Geometry: final body of the model. Coordinates: model frame, mm. A direction names the side the tool comes from. Coordinates: 2 decimals unless noted, no trailing zeros. Order: outer loops, then holes, each group sorted by start corner. A loop starts at its lowest first (then second) coordinate and runs counter-clockwise, first axis right, second up. Notation, with made-up numbers: M -24.5,2.5 L -20.5,2.5 A9 ccw -20.5,17.5 Z; hole C 85,63 d3. An arc over 180 degrees is marked long. Write item = value, one per line. Start each with the question number.
```python
from build123d import *

# Parameters (mm, degrees)
F1_DEPTH = 6.223
F3_DEPTH = 25.4
F4_R     = 5.08
F5_R     = 7.62


with BuildPart() as f1:
    # F0 (on Top) → F1 (new body)
    with BuildSketch(Plane.XY):
        Polygon((-38.1, 0), (0, 0), (38.1, 0), (38.1, 9.5885), (44.45, 9.5885), (44.45, 12.7), (44.45, 15.8115), (38.1, 15.8115), (38.1, 41.3385), (44.45, 41.3385), (44.45, 44.45), (44.45, 47.5615), (38.1, 47.5615), (38.1, 57.15), (0, 57.15), (-38.1, 57.15), (-38.1, 47.5615), (-44.45, 47.5615), (-44.45, 44.45), (-44.45, 41.3385), (-38.1, 41.3385), (-38.1, 15.8115), (-44.45, 15.8115), (-44.45, 12.7), (-44.45, 9.5885), (-38.1, 9.5885), align=None)
    extrude(amount=F1_DEPTH)

    # F2 (on face) → F3 (cut)
    with BuildSketch(Plane.XY.offset(6.223)):
        Polygon((-28.575, 46.0375), (-28.575, 11.1125), (-5.291667, 28.575), align=None)
        Polygon((-24.341667, 50.8), (0, 32.54375), (24.341667, 50.8), align=None)
        Polygon((28.575, 46.0375), (5.291667, 28.575), (28.575, 11.1125), align=None)
        Polygon((24.341667, 6.35), (0, 24.60625), (-24.341667, 6.35), align=None)
    extrude(amount=-F3_DEPTH, mode=Mode.SUBTRACT)

    # F4
    f4_edges = [f1.edges().sort_by_distance(p)[0] for p in [
        (-28.575, 11.1125, 3.1115),
        (-28.575, 46.0375, 3.1115),
        (-5.291667, 28.575, 3.1115),
        (24.341667, 6.35, 3.1115),
        (0, 24.60625, 3.1115),
        (-24.341667, 6.35, 3.1115),
        (28.575, 11.1125, 3.1115),
        (28.575, 46.0375, 3.1115),
        (5.291667, 28.575, 3.1115),
        (0, 32.54375, 3.1115),
        (24.341667, 50.8, 3.1115),
        (-24.341667, 50.8, 3.1115),
    ]]
    fillet(f4_edges, radius=F4_R)

    # F5
    f5_edges = [f1.edges().sort_by_distance(p)[0] for p in [
        (-38.1, 57.15, 3.1115),
        (38.1, 57.15, 3.1115),
        (38.1, 0, 3.1115),
        (-38.1, 0, 3.1115),
    ]]
    fillet(f5_edges, radius=F5_R)


solid = f1.part
```
Item 1: Section query C-C on x = -24. Output: boundary loops of the cut face in (y, z), and give its area (3 significant figures).
Item 2: Reachability of faces 1 (the flat face through (38.1, 28, 3)), 2 (the flat face through (41, 47.562, 3)), 3 (the cylindrical face through (-8.68, 28.51, 3.07)) from +Z, -Z, +X, -X, +Y, -Y: full face, straight path, thin tool, end or side. Return the list, or none.
Item 3: Section query A-A on x = 1.5. Output: boundary loops of the cut face in (y, z), and give its area (3 significant figures).
Item 4: Draft query along X for faces 4 (the cylindrical face through (35.809, 2.173, 3.155)), 5 (the flat face through (41, 9.588, 3)), 6 (the cylindrical face through (0.046, 23.336, 3.068)). Return one class per face: pulls with the +X half, pulls with the -X half, needs draft (parallel to the pull), parting line crosses it, or undercut.
Item 5: Section query D-D on y = 19. Output: boundary loops of the cut face in (x, z) (3 decimals).
Item 6: Material intervals for probe 1 along Y at (x, z) = (-41, 0.5); probe 2 along Y at (x, z) = (2, 3.75); probe 3 along Y at (x, z) = (10, 0.75), sorted ascending. Write a range as [from, to].
Item 7: Section query B-B on y = 30. Output: boundary loops of the cut face in (x, z) (3 decimals), and give its area (3 significant figures).
Item 8: First-contact query: pin 1 (1.5 mm diameter, centred on y = 40.5, z = 1.5, fed in from +X); pin 2 (3 mm diameter, centred on x = -41.5, z = 3, fed in from -Y); pin 3 (3 mm diameter, centred on y = 30.5, z = 3.5, fed in from -X). Flat tips, straight axial feed; report the tip coordinate or a pass-through.
Ans:
q1.outline = M 0,0 L 16.22,0 L 16.22,6.22 L 0,6.22 Z; M 40.93,0 L 57.15,0 L 57.15,6.22 L 40.93,6.22 Z
q1.area = 202 mm^2
q2.face_1 = +Z, -Z, +X
q2.face_2 = +Z, -Z, +X, +Y
q2.face_3 = +Z, -Z
q3.outline = M 0,0 L 6.35,0 L 6.35,6.22 L 0,6.22 Z; M 23.11,0 L 34.04,0 L 34.04,6.22 L 23.11,6.22 Z; M 50.8,0 L 57.15,0 L 57.15,6.22 L 50.8,6.22 Z
q3.area = 147 mm^2
q4.face_4 = pulls with the +X half
q4.face_5 = needs draft
q4.face_6 = undercut
q5.outline = M -38.1,0 L -28.038,0 L -28.038,6.223 L -38.1,6.223 Z; M -18.058,0 L -7.475,0 L -7.475,6.223 L -18.058,6.223 Z; M 7.475,0 L 18.058,0 L 18.058,6.223 L 7.475,6.223 Z; M 28.038,0 L 38.1,0 L 38.1,6.223 L 28.038,6.223 Z
q6.probe_1 = [9.59, 15.81], [41.34, 47.56]
q6.probe_2 = [0, 6.35], [22.93, 34.22], [50.8, 57.15]
q6.probe_3 = [0, 6.43], [17.11, 25.16], [31.99, 40.04], [50.72, 57.15]
q7.outline = M -38.1,0 L -28.575,0 L -28.575,6.223 L -38.1,6.223 Z; M -8.882,0 L 8.882,0 L 8.882,6.223 L -8.882,6.223 Z; M 28.575,0 L 38.1,0 L 38.1,6.223 L 28.575,6.223 Z
q7.area = 229 mm^2
q8.pin_1 = 38.1
q8.pin_2 = 9.59
q8.pin_3 = -38.1
